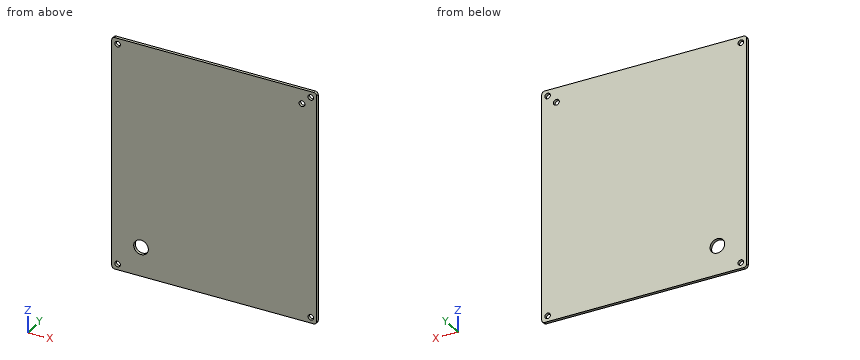
from build123d import *

# Parameters (mm, degrees)
SKETCH1_W           = 140
SKETCH1_H           = 160
BOSS_EXTRUDE1_DEPTH = 2
SKETCH2_R           = 1.9
SKETCH2_R_2         = 2
SKETCH2_R_3         = 5
CUT_EXTRUDE1_DEPTH  = 10
FILLET1_R           = 2


with BuildPart() as part:
    # Sketch1 → Boss-Extrude1 (new body)
    with BuildSketch(Plane(origin=(0, 0, 0), x_dir=(1, 0, 0), z_dir=(0, 1, 0))):
        with Locations((70, 80)):
            Rectangle(SKETCH1_W, SKETCH1_H)
    extrude(amount=BOSS_EXTRUDE1_DEPTH)

    # Sketch2 → Cut-Extrude1 (cut)
    with BuildSketch(Plane(origin=(0, 2, 0), x_dir=(1, 0, 0), z_dir=(0, 1, 0))):
        with Locations(Location((4, 156, 0), (0, 0, 270))):
            Circle(SKETCH2_R)
        with Locations(Location((136, 156, 0), (0, 0, 90))):
            Circle(SKETCH2_R)
        with Locations(Location((136, 4, 0), (0, 0, 270))):
            Circle(SKETCH2_R)
        with Locations(Location((4, 4, 0), (0, 0, 90))):
            Circle(SKETCH2_R)
        with Locations(Location((130, 10, 0), (0, 0, 270))):
            Circle(SKETCH2_R_2)
        with Locations(Location((20, 140, 0), (0, 0, 270))):
            Circle(SKETCH2_R_3)
    extrude(amount=-CUT_EXTRUDE1_DEPTH, mode=Mode.SUBTRACT)

    # Fillet1
    fillet1_edges = [part.edges().sort_by_distance(p)[0] for p in [
        (0, 1, -160),
        (140, 1, -160),
        (140, 1, 0),
        (0, 1, 0),
    ]]
    fillet(fillet1_edges, radius=FILLET1_R)


solid = part.part
Can you work these out from the model? Positions are in its coordinate system, mm. Give positions to 0.01 mm unless a question says otherwise; leave off trailing zeros. Loops run counter-clockwise (first coordinate to the right, second up) from the corner with the lowest first, then second, coordinate; pieces in that order, holes last. Notation, with made-up numbers: M 54,35 L 108,35 A22 ccw 108,41 Z; hole C -32,10 d4. An arc over 180 degrees is marked long. One line per item, written item: value.
1) I'm going to push a flat-ended pin straight in: pin 1 (3 mm diameter, centred on x = 136, z = -156, fed in from +Y). Where does the tip first touch, or does it pass through?
Geometry check:
pin 1: passes through
2) Imagine slicing it at B-B on x = 20. Write out the boundary of the cut face in (y, z), and give its area (3 significant figures).
Geometry check:
outline: M 0,-160 L 2,-160 L 2,-145 L 0,-145 Z; M 0,-135 L 2,-135 L 2,0 L 0,0 Z
area: 300 mm²
3) Imagine slicing it at C-C on x = 4. Write out the boundary of the cut face in (y, z), and give its area (3 significant figures).
Geometry check:
outline: M 0,-160 L 2,-160 L 2,-157.9 L 0,-157.9 Z; M 0,-154.1 L 2,-154.1 L 2,-5.9 L 0,-5.9 Z; M 0,-2.1 L 2,-2.1 L 2,0 L 0,0 Z
area: 305 mm²
4) Please list where these lines run through material, in increasing order: line 1 (X direction, y = 0.65, z = -4); line 2 (Z direction, x = 136, y = 0.5); line 3 (X direction, y = 1.1, z = -10).
Geometry check:
line 1: x = 0 to 2.1, 5.9 to 134.1, 137.9 to 140
line 2: z = -160 to -157.9, -154.1 to -5.9, -2.1 to 0
line 3: x = 0 to 128, 132 to 140
5) Imagine slicing it at A-A on z = -10. Write out the boundary of the cut face in (x, y), and give its area (3 significant figures).
Geometry check:
outline: M 0,0 L 128,0 L 128,2 L 0,2 Z; M 132,0 L 140,0 L 140,2 L 132,2 Z
area: 272 mm²
